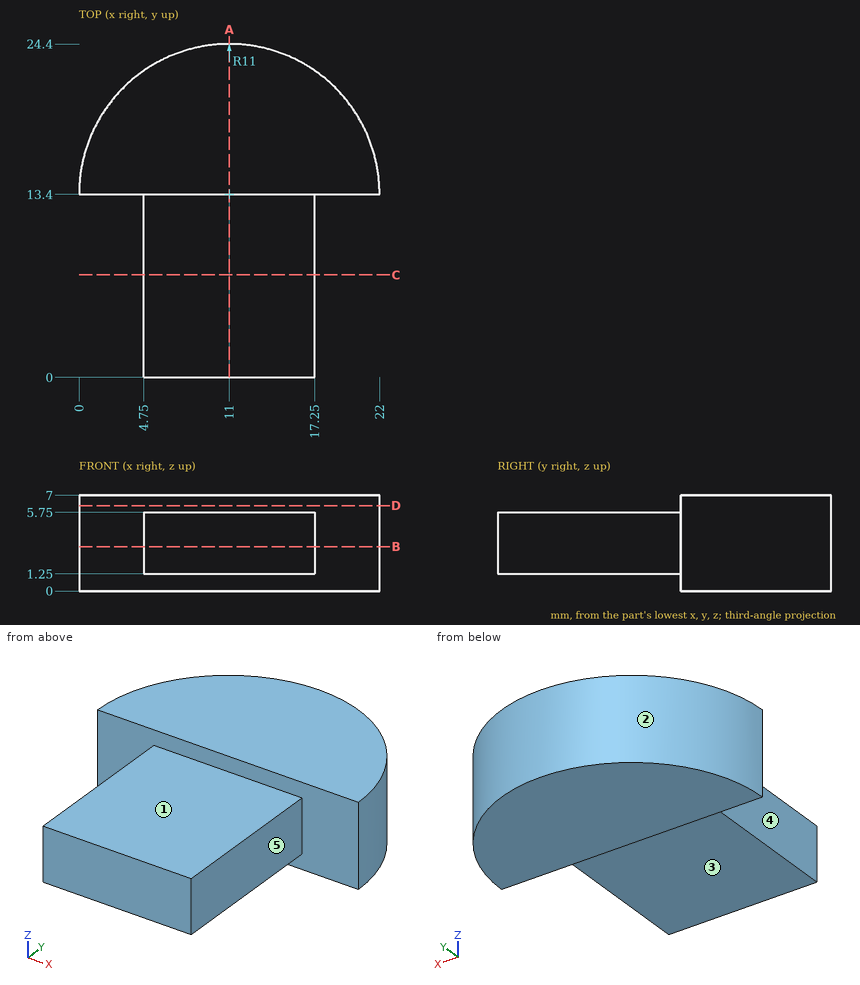
Verification items for this drawing (mm, ordinates from the low corner). A direction names the side the tool comes from. Coordinates: 2 decimals unless noted, no trailing zeros. Order: outer loops, then holes, each group sorted by start corner. A loop starts at its lowest first (then second) coordinate and runs counter-clockwise, first axis right, second up. Notation, with made-up numbers: (41.5, 39) -> (95.5, 39) arc R5 cw to (95.5, 44) -> close; hole circle Ø6 at (47.25, 20.25). An arc over 180 degrees is marked (long way). Answer as CSV lines item,"result". Start each with the question number.
1) Cross-section at C-C, the plane y = 7.5. Record the boundary of the cut face in (x, z), then the cut area to 4 significant figures.
2) Cross-section at A-A, the plane x = 11. Record the boundary of the cut face in (y, z), then the cut area to 3 significant figures.
3) Cross-section at B-B, the plane z = 3.25. Record the boundary of the cut face in (x, y).
4) Material ranges on L1, parallel to X at y = 4.75, z = 2.75; L2, parallel to Z at x = 8.5, y = 4; L3, parallel to X at y = 13.5, z = 6, recorded low to high. Write a range as [from, to].
5) Set-up check for the marked faces 1, 2, 3, 4 and 5: record each of +Z, -Z, +X, -X, +Y, -Y from which the full face is reachable in a straight line by a thin tool's end or side.
6) Gauge pin test, flat ends, axial feed: pin 1 Ø3.5 at (y, z) = (7, 4.5) entering from +X; pin 2 Ø1.5 at (x, y) = (2.5, 7.5) entering from +Z; pin 3 Ø1 at (y, z) = (15, 1) entering from +X; pin 4 Ø3.5 at (y, z) = (8.5, 4) entering from -X. Record the tip position at first contact, or that the pin passes through.
7) Cross-section at D-D, the plane z = 6.25. Record the boundary of the cut face in (x, y).
Conclusion:
1,outline,"(4.75, 1.25) -> (17.25, 1.25) -> (17.25, 5.75) -> (4.75, 5.75) -> close"
1,area,"56.25 mm²"
2,outline,"(0, 1.25) -> (13.4, 1.25) -> (13.4, 0) -> (24.4, 0) -> (24.4, 7) -> (13.4, 7) -> (13.4, 5.75) -> (0, 5.75) -> close"
2,area,"137 mm²"
3,outline,"(0, 13.4) -> (4.75, 13.4) -> (4.75, 0) -> (17.25, 0) -> (17.25, 13.4) -> (22, 13.4) arc R11 ccw to start"
4,L1,"x = [4.75, 17.25]"
4,L2,"z = [1.25, 5.75]"
4,L3,"x = [0, 22]"
5,face 1,"+Z, +X, -X, -Y"
5,face 2,"+Z, -Z, +Y"
5,face 3,"-Z, +X, -X, -Y"
5,face 4,"+Z, -Z, -X, -Y"
5,face 5,"+Z, -Z, +X, -Y"
6,pin 1,"stops at x = 17.25"
6,pin 2,"passes through"
6,pin 3,"stops at x = 21.94"
6,pin 4,"stops at x = 4.75"
7,outline,"(0, 13.4) -> (22, 13.4) arc R11 ccw to start"
